Geometry check sheet. Reference: the model listing, model coordinates, mm. Face numbers are marked on the shaded views. A direction names the side the tool comes from. Coordinates: 2 decimals unless noted, no trailing zeros. Order: outer loops, then holes, each group sorted by start corner. A loop starts at its lowest first (then second) coordinate and runs counter-clockwise, first axis right, second up. Notation, with made-up numbers: (43.25, 42) - (75.25, 42) arc R20 cw to (75.25, 81) - close; hole circle Ø3 at (30, -34). An arc over 180 degrees is marked (long way). Use CSV: the item, a comma, the result in double quotes. Start each with the question number.
1) Sectioned sample at D-D, the plane x = 8. Record the cut outline in (y, z), and give its area (3 significant figures).
2) Depth check by flat-ended pin: P1, Ø1.5, axis at x = -1, z = 13.5, coming from the +Y side; P2, Ø1.5, axis at x = 1.5, z = 6, coming from the +Y side; P3, Ø2, axis at x = 6, y = -2, coming from the +Z side. Enter the tip coordinate at first touch or a pass-through.
3) Sectioned sample at C-C, the plane x = -2. Record the cut outline in (y, z).
4) Tool access check on the marked faces 4, 5 and 6. Record the directions out of +Z, -Z, +X, -X, +Y, -Y that give a thin tool (end or side, any length) a straight path to the whole face; none if there is none.
5) Sectioned sample at B-B, the plane y = 1.5. Record the cut outline in (x, z).
6) Sectioned sample at A-A, the plane z = 2.75. Record the cut outline in (x, y).
7) Draft check along X on the marked faces 1, 2 and 3. Enter one of: released by +X, released by -X, zero draft, split by the parting line, or undercut.
8) Thickness scan on probe 1 along Y at (x, z) = (0, 6.5); probe 2 along Y at (x, z) = (-8, 10.5); probe 3 along Z at (x, y) = (9.5, 0.25). Record the ranges inside material, lowest first. Write a range as [from, to].
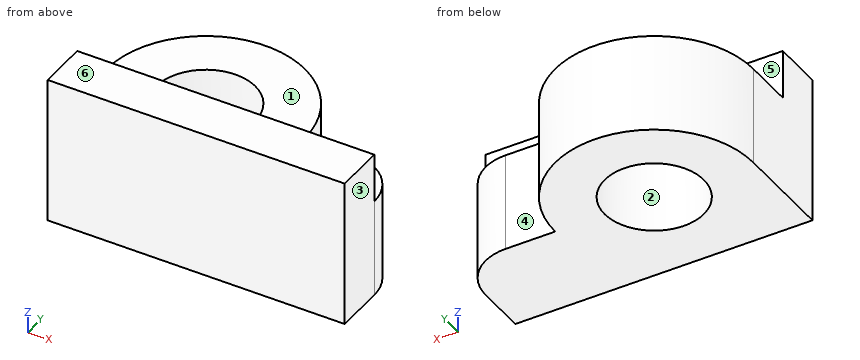
from build123d import *

# Parameters (mm, degrees)
SKETCH_1_R      = 5
EXTRUDE_1_DEPTH = 10
EXTRUDE_2_DEPTH = 15


with BuildPart() as part:
    # 草圖1 → 填料-伸長1 (new body)
    with BuildSketch(Plane.XY):
        with BuildLine():
            Line((-10, 0), (-10, -10))
            Line((-10, -10), (20, -10))
            Line((20, -10), (20, -5))
            ThreePointArc((20, -5), (18.535533906, -1.464466094), (15, 0))
            Line((15, 0), (10, 0))
            ThreePointArc((10, 0), (0, 10), (-10, 0))
        make_face()
        Circle(SKETCH_1_R, mode=Mode.SUBTRACT)
    extrude(amount=EXTRUDE_1_DEPTH)

    # 草圖1<3> → 填料-伸長2 (add)
    with BuildSketch(Plane.XY):
        Polygon((0, -5), (-10, -5), (-10, -10), (20, -10), (20, -5), align=None)
    extrude(amount=EXTRUDE_2_DEPTH)


solid = part.part
Evaluation:
1,outline,"(-10, 0) - (6, 0) - (6, 10) - (-5, 10) - (-5, 15) - (-10, 15) - close"
1,area,"185 mm²"
2,P1,"y = -5"
2,P2,"y = 9.97"
2,P3,"z = 10"
3,outline,"(-10, 0) - (-4.58, 0) - (-4.58, 10) - (-5, 10) - (-5, 15) - (-10, 15) - close; (4.58, 0) - (9.8, 0) - (9.8, 10) - (4.58, 10) - close"
4,face 4,"+Z, -Z, +X, +Y"
4,face 5,"+Z, +X, -X, +Y"
4,face 6,"+Z, +X, -X, +Y, -Y"
5,outline,"(-9.89, 0) - (-4.77, 0) - (-4.77, 10) - (-9.89, 10) - close; (4.77, 0) - (9.89, 0) - (9.89, 10) - (4.77, 10) - close"
6,outline,"(-10, -10) - (20, -10) - (20, -5) arc R5 ccw to (15, 0) - (10, 0) arc R10 ccw to (-10, 0) - close; hole circle Ø10 at (0, 0)"
7,face 1,"zero draft"
7,face 2,"undercut"
7,face 3,"released by +X"
8,probe 1,"[-10, -5], [5, 10]"
8,probe 2,"[-10, -5]"
8,probe 3,"[0, 10]"
